```python
from build123d import *

# Parameters (mm, degrees)
F0_W     = 7.62
F0_H     = 50.8
F1_DEPTH = 2.1844
F3_DEPTH = 16.51
F4_W     = 2.794
F4_H     = 1.5748
F4_W_2   = 2.9464
F4_W_3   = 1.7272
F5_DEPTH = 0.3683
F6_W     = 2.032
F6_H     = 0.508
F7_DEPTH = 0.3302
F9_DEPTH = 25.4


with BuildPart() as f1:
    # F0 (on Top) → F1 (new body)
    with BuildSketch(Plane.XY):
        Rectangle(F0_W, F0_H)
    extrude(amount=F1_DEPTH)

    # F2 (on Front) → F3 (cut, symmetric)
    with BuildSketch(Plane.XZ):
        Polygon((-0.9652, 0), (1.27, 0), (1.27, 2.1844), (-1.27, 2.1844), (-1.27, 1.4732), (-0.9652, 1.4732), align=None)
    extrude(amount=F3_DEPTH, both=True, mode=Mode.SUBTRACT)

    # F4 (on face) → F5 (join)
    with BuildSketch(Plane(origin=(1.27, 0, 0), x_dir=(0, -1, 0), z_dir=(-1, 0, 0))):
        with Locations((0, 0.7874)):
            Rectangle(F4_W, F4_H)
        with Locations((-8.2042, 0.7874)):
            Rectangle(F4_W_2, F4_H)
        with Locations((8.2042, 0.7874)):
            Rectangle(F4_W_2, F4_H)
        with Locations((-15.6464, 0.7874)):
            Rectangle(F4_W_3, F4_H)
        with Locations((15.6464, 0.7874)):
            Rectangle(F4_W_3, F4_H)
    extrude(amount=F5_DEPTH)

    # F6 (on face) → F7 (join)
    with BuildSketch(Plane.YZ.offset(-0.9652)):
        with Locations((-4.064, 1.016)):
            Rectangle(F6_W, F6_H)
        with Locations((4.064, 1.016)):
            Rectangle(F6_W, F6_H)
        with Locations((-12.192, 1.016)):
            Rectangle(F6_W, F6_H)
        with Locations((12.192, 1.016)):
            Rectangle(F6_W, F6_H)
    extrude(amount=F7_DEPTH)

    # F8 (on face) → F9 (cut)
    with BuildSketch(Plane.XY.offset(2.1844)):
        Polygon((-3.100628, 22.160923), (-1.27, 16.51), (1.27, 16.51), (1.27, 22.160923), align=None)
        Polygon((1.27, -16.51), (-1.27, -16.51), (-3.100628, -22.160923), (1.27, -22.160923), align=None)
    extrude(amount=-F9_DEPTH, mode=Mode.SUBTRACT)


with BuildPart() as f10_1:
    # F10: copy of F1
    add(f1.part.moved(Location((7.62, 0, 0))))


with BuildPart() as f11_1:
    # F11: copy of F10_1
    add(f10_1.part.moved(Location((7.62, 0, 0))))


with BuildPart() as f12_1:
    # F12: copy of F11_1
    add(f11_1.part.moved(Location((7.62, 0, 0))))


solid = f1.part
```
Verification items for the finished model (mm, model axes). A direction names the side the tool comes from. Give positions to 0.01 mm unless a question says otherwise; leave off trailing zeros. Order: outer loops, then holes, each group sorted by start corner. A loop starts at its lowest first (then second) coordinate and runs counter-clockwise, first axis right, second up. Notation, with made-up numbers: M 1.25,8.5 L 12.25,8.5 A22 cw 12.25,22.5 Z; hole C 9.25,52.25 d8. An arc over 180 degrees is marked long. Answer in a Markdown table with one row per item. Add a question column.
Item 1: Section check C-C, the plane y = 16. Enter the section's corners in (x, z).
Item 2: Section check B-B, the plane x = -1.75. Enter the section's corners in (y, z).
Item 3: Section check A-A, the plane y = -4. Enter the section's corners in (x, z) (3 decimals).
Item 4: Scan lines: probe 1 along Y at (x, z) = (-1, 0.45); probe 2 along X at (y, z) = (-4, 1) (3 decimals); probe 3 along X at (y, z) = (-15.5, 1.2). Record each from-to range of solid material in increasing order. Write a range as from..to.
Item 5: Mould release check, pull along Y, two halves, no side actions. Record for faces 4 (the flat face through (0, 25.4, 1)), 5 (the flat face through (2, 0, 0)), 6 (the flat face through (0.902, -16, 1)): released by +Y, released by -Y, zero draft, split by the parting line, or undercut.
Item 6: Tool access check on faces 1 (the flat face through (1.27, 0, 2)), 2 (the flat face through (3.81, 0, 1)), 3 (the flat face through (-1, -22.161, 1)). Record the directions out of +Z, -Z, +X, -X, +Y, -Y that give a thin tool (end or side, any length) a straight path to the whole face; none if there is none.
Filled sheet:
| question | item | result |
|---|---|---|
| 1 | outline | M -3.81,0 L -0.97,0 L -0.97,1.47 L -1.27,1.47 L -1.27,2.18 L -3.81,2.18 Z; M 0.9,0 L 3.81,0 L 3.81,2.18 L 1.27,2.18 L 1.27,1.57 L 0.9,1.57 Z |
| 2 | outline | M -25.4,0 L -22.16,0 L -22.16,2.18 L -25.4,2.18 Z; M -17.99,0 L 17.99,0 L 17.99,2.18 L -17.99,2.18 Z; M 22.16,0 L 25.4,0 L 25.4,2.18 L 22.16,2.18 Z |
| 3 | outline | M -3.81,0 L -0.965,0 L -0.965,0.762 L -0.635,0.762 L -0.635,1.27 L -0.965,1.27 L -0.965,1.473 L -1.27,1.473 L -1.27,2.184 L -3.81,2.184 Z; M 1.27,0 L 3.81,0 L 3.81,2.184 L 1.27,2.184 Z |
| 4 | probe 1 | y = -25.4..-22.16, -16.51..16.51, 22.16..25.4 |
| 4 | probe 2 | x = -3.81..-0.635, 1.27..3.81 |
| 4 | probe 3 | x = -3.81..-0.97, 0.9..3.81 |
| 5 | face 4 | released by +Y |
| 5 | face 5 | zero draft |
| 5 | face 6 | undercut |
| 6 | face 1 | +Z |
| 6 | face 2 | +Z, -Z, +X, +Y, -Y |
| 6 | face 3 | +Z, -Z |
